Could you check a few things on this model? Use its own coordinates, in mm. A direction names the side the tool comes from. Coordinates: 2 decimals unless noted, no trailing zeros. Order: outer loops, then holes, each group sorted by start corner. A loop starts at its lowest first (then second) coordinate and runs counter-clockwise, first axis right, second up. Notation, with made-up numbers: (-2.5, 72) - (30.5, 72) arc R18 cw to (30.5, 103) - close; hole circle Ø1 at (64.5, 19.25). An arc over 180 degrees is marked (long way). Answer as CSV lines item,"result". Start each with the question number.
1. Thinking about a two-plate mould opening in Z: for faces 1 (the face through (-16, 5, 35.5)), 2 (the face through (42, 4, 31.5)), 3 (the face through (3, 18.114, 17)), which applies, released by +Z, released by -Z, zero draft, split by the parting line, or undercut?
2. For pin 1 (20 mm diameter, centred on x = 12.63, z = 26.5, fed in from +Y); pin 2 (1.5 mm diameter, centred on x = 9.5, z = 43, fed in from -Y); pin 3 (1.5 mm diameter, centred on y = 7, z = 6.5, fed in from -X); pin 4 (2.5 mm diameter, centred on x = 41, y = 4, fed in from +Z), each with a flat end and sliding along its axis, tell me the tip position at first contact or that it passes through.
3. I want a section at D-D, the plane y = 6. List the corners of the cut face in (x, z) for me.
4. For faces 4 (the face through (-16, -13.828, 13)), 5 (the face through (-16, 5, 15.5)), 6 (the face through (42, 4, 36.5)), which set-ups out of +Z, -Z, +X, -X, +Y, -Y let a thin tool reach every point of the face, with its end or its side?
5. I need wall thicknesses on probe 1 along X at (y, z) = (3, 18); probe 2 along X at (y, z) = (14.5, 16); probe 3 along Z at (x, y) = (-16, 20). Which ranges of each line are inside material? Lowest first, please.
6. I want a section at B-B, the plane z = 26.5. List the corners of the cut face in (x, y) for me.
7. I want a section at A-A, the plane y = 0. List the corners of the cut face in (x, z) for me, and give its area (3 significant figures).
8. I want a section at C-C, the plane x = 27. List the corners of the cut face in (y, z) for me, and give its area (4 significant figures).
from build123d import *

# Parameters (mm, degrees)
BOSS_EXTRUDE4_DEPTH = 48
SKETCH2_W           = 43
SKETCH2_H           = 43
CUT_EXTRUDE2_DEPTH  = 43
SKETCH5_R           = 11.15
CUT_EXTRUDE3_DEPTH  = 2.5
SKETCH7_R           = 3
CUT_EXTRUDE4_DEPTH  = 2.5
CUT_EXTRUDE5_DEPTH  = 5
SKETCH9_W           = 36.942088093
SKETCH9_H           = 5
BOSS_EXTRUDE5_DEPTH = 5
SKETCH12_W          = 36.942088093
SKETCH12_H          = 5
BOSS_EXTRUDE6_DEPTH = 5


with BuildPart() as part:
    # Sketch1 → Boss-Extrude4 (new body)
    with BuildSketch(Plane(origin=(0, 0, 0), x_dir=(0, 1, 0), z_dir=(0, 0, 1))):
        Polygon((3.614394585, 8.871473005), (-15.885605415, 8.871473005), (-15.885605415, 13.871473005), (23.114394585, 13.871473005), (23.114394585, -39.128526995), (-15.885605415, -39.128526995), (-15.885605415, -34.128526995), (3.614394585, -34.128526995), align=None)
    extrude(amount=BOSS_EXTRUDE4_DEPTH)

    # Sketch2 → Cut-Extrude2 (cut)
    with BuildSketch(Plane.XY.offset(48)):
        with Locations((12.628526995, -3.385605415)):
            Rectangle(SKETCH2_W, SKETCH2_H)
    extrude(amount=-CUT_EXTRUDE2_DEPTH, mode=Mode.SUBTRACT)

    # Sketch5 → Cut-Extrude3 (cut)
    with BuildSketch(Plane.XZ.offset(-18.114394585)):
        with Locations(Location((12.628526995, 26.5, 0), (0, 0, 270))):
            Circle(SKETCH5_R)
    extrude(amount=-CUT_EXTRUDE3_DEPTH, mode=Mode.SUBTRACT)

    # Sketch7 → Cut-Extrude4 (cut)
    with BuildSketch(Plane.XZ.offset(-20.614394585)):
        with Locations(Location((12.628526995, 26.5, 0), (0, 0, 270))):
            Circle(SKETCH7_R)
    extrude(amount=-CUT_EXTRUDE4_DEPTH, mode=Mode.SUBTRACT)

    # Sketch8 → Cut-Extrude5 (cut)
    with BuildSketch(Plane.XZ.offset(-18.114394585)):
        with BuildLine():
            Line((-4, 43.474351547), (0, 43.474351547))
            ThreePointArc((0, 43.474351547), (2.15, 41.324351547), (0, 39.174351547))
            Line((0, 39.174351547), (-4, 39.174351547))
            ThreePointArc((-4, 39.174351547), (-6.15, 41.324351547), (-4, 43.474351547))
        make_face()
        with BuildLine():
            Line((28.856423603, 12.390432875), (24.856423603, 12.390432875))
            ThreePointArc((24.856423603, 12.390432875), (22.706423603, 10.240432875), (24.856423603, 8.090432875))
            Line((24.856423603, 8.090432875), (28.856423603, 8.090432875))
            ThreePointArc((28.856423603, 8.090432875), (31.006423603, 10.240432875), (28.856423603, 12.390432875))
        make_face()
        with BuildLine():
            Line((29.25705399, 43.474351547), (25.25705399, 43.474351547))
            ThreePointArc((25.25705399, 43.474351547), (23.10705399, 41.324351547), (25.25705399, 39.174351547))
            Line((25.25705399, 39.174351547), (29.25705399, 39.174351547))
            ThreePointArc((29.25705399, 39.174351547), (31.40705399, 41.324351547), (29.25705399, 43.474351547))
        make_face()
        with BuildLine():
            Line((-3.599369613, 12.390432875), (0.400630387, 12.390432875))
            ThreePointArc((0.400630387, 12.390432875), (2.550630387, 10.240432875), (0.400630387, 8.090432875))
            Line((0.400630387, 8.090432875), (-3.599369613, 8.090432875))
            ThreePointArc((-3.599369613, 8.090432875), (-5.749369613, 10.240432875), (-3.599369613, 12.390432875))
        make_face()
    extrude(amount=-CUT_EXTRUDE5_DEPTH, mode=Mode.SUBTRACT)

    # Sketch9 → Boss-Extrude5 (add)
    with BuildSketch(Plane(origin=(-13.871473005, 0, 0), x_dir=(0, -1, 0), z_dir=(-1, 0, 0))):
        with Locations((-4.643350539, 33)):
            Rectangle(SKETCH9_W, SKETCH9_H)
        with Locations((-4.643350539, 13)):
            Rectangle(SKETCH9_W, SKETCH9_H)
    extrude(amount=BOSS_EXTRUDE5_DEPTH)

    # Sketch12 → Boss-Extrude6 (add)
    with BuildSketch(Plane.YZ.offset(39.128526995)):
        with Locations((4.643350539, 34)):
            Rectangle(SKETCH12_W, SKETCH12_H)
        with Locations((4.643350539, 14)):
            Rectangle(SKETCH12_W, SKETCH12_H)
    extrude(amount=BOSS_EXTRUDE6_DEPTH)


solid = part.part
Solved:
1,face 1,"released by +Z"
1,face 2,"undercut"
1,face 3,"zero draft"
2,pin 1,"stops at y = 23.11"
2,pin 2,"stops at y = 18.11"
2,pin 3,"stops at x = -13.87"
2,pin 4,"stops at z = 36.5"
3,outline,"(-18.87, 10.5) - (-13.87, 10.5) - (-13.87, 0) - (39.13, 0) - (39.13, 11.5) - (44.13, 11.5) - (44.13, 16.5) - (39.13, 16.5) - (39.13, 31.5) - (44.13, 31.5) - (44.13, 36.5) - (39.13, 36.5) - (39.13, 48) - (34.13, 48) - (34.13, 5) - (-8.87, 5) - (-8.87, 48) - (-13.87, 48) - (-13.87, 35.5) - (-18.87, 35.5) - (-18.87, 30.5) - (-13.87, 30.5) - (-13.87, 15.5) - (-18.87, 15.5) - close"
4,face 4,"+Z, -Z, -X, -Y"
4,face 5,"-X, +Y, -Y"
4,face 6,"+Z, +X, +Y, -Y"
5,probe 1,"x = -13.87 to -8.87, 34.13 to 39.13"
5,probe 2,"x = -13.87 to -8.87, 34.13 to 44.13"
5,probe 3,"z = 10.5 to 15.5, 30.5 to 35.5"
6,outline,"(-13.87, -15.89) - (-8.87, -15.89) - (-8.87, 18.11) - (1.48, 18.11) - (1.48, 20.61) - (9.63, 20.61) - (9.63, 23.11) - (-13.87, 23.11) - close; (15.63, 20.61) - (23.78, 20.61) - (23.78, 18.11) - (34.13, 18.11) - (34.13, -15.89) - (39.13, -15.89) - (39.13, 23.11) - (15.63, 23.11) - close"
7,outline,"(-18.87, 10.5) - (-13.87, 10.5) - (-13.87, 0) - (-8.87, 0) - (-8.87, 48) - (-13.87, 48) - (-13.87, 35.5) - (-18.87, 35.5) - (-18.87, 30.5) - (-13.87, 30.5) - (-13.87, 15.5) - (-18.87, 15.5) - close; (34.13, 0) - (39.13, 0) - (39.13, 11.5) - (44.13, 11.5) - (44.13, 16.5) - (39.13, 16.5) - (39.13, 31.5) - (44.13, 31.5) - (44.13, 36.5) - (39.13, 36.5) - (39.13, 48) - (34.13, 48) - close"
7,area,"580 mm2"
8,outline,"(3.61, 0) - (23.11, 0) - (23.11, 8.09) - (18.11, 8.09) - (18.11, 5) - (3.61, 5) - close; (18.11, 12.39) - (23.11, 12.39) - (23.11, 39.17) - (18.11, 39.17) - close; (18.11, 43.47) - (23.11, 43.47) - (23.11, 48) - (18.11, 48) - close"
8,area,"269.5 mm2"
